Geometry check sheet. Reference: the model listing, model coordinates, mm. Face numbers are marked on the shaded views. A direction names the side the tool comes from. Coordinates: 2 decimals unless noted, no trailing zeros. Order: outer loops, then holes, each group sorted by start corner. A loop starts at its lowest first (then second) coordinate and runs counter-clockwise, first axis right, second up. Notation, with made-up numbers: (-22, 66) - (30, 66) arc R10 ccw to (30, 82) - close; hole circle Ø11 at (75, 57). An arc over 180 degrees is marked (long way). Return JSON: item names as keys, results as strings. Group by question number.
Item 1: Section check B-B on z = 51. Give the number of separate pieces and of enclosed holes in the cut face, then the cut area to 3 significant figures.
Item 2: Tool access check on the marked faces 1 and 2. Record the directions out of +Z, -Z, +X, -X, +Y, -Y that give a thin tool (end or side, any length) a straight path to the whole face; none if there is none.
Item 3: Section check A-A on y = 16.5. Enter the section's corners in (x, z) (3 decimals).
Item 4: Gauge pin test, flat ends, axial feed: pin 1 (1.6 mm diameter, centred on x = 36.5, y = 30, fed in from +Z); pin 2 (2.5 mm diameter, centred on x = 36.5, y = -8, fed in from +Z); pin 3 (1.5 mm diameter, centred on x = 8, y = -9.5, fed in from +Z) (3 decimals). Record the tip position at first contact, or that the pin passes through.
Item 5: Scan lines: probe 1 along X at (y, z) = (0.5, 11.5) (3 decimals); probe 2 along Z at (x, y) = (-19, -13) (3 decimals). Record each from-to range of solid material in increasing order.
Item 6: Section check C-C on x = -25.5. Enter the section's corners in (y, z) (3 decimals), then the cut area to 3 significant figures.
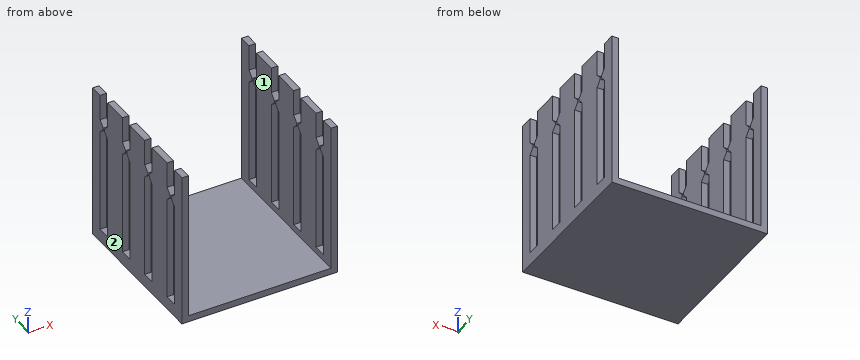
from build123d import *

# Parameters (mm, degrees)
F0_W     = 76.2
F0_H     = 76.2
F1_DEPTH = 76.2
F3_DEPTH = 131.88104
F4_W     = 69.85
F4_H     = 73.025
F5_DEPTH = 151.50575


with BuildPart() as f1:
    # F0 (on Top) → F1 (new body)
    with BuildSketch(Plane.XY):
        Rectangle(F0_W, F0_H)
    extrude(amount=F1_DEPTH)

    # F2 (on face) → F3 (cut)
    with BuildSketch(Plane.YZ.offset(38.1)):
        with BuildLine():
            Line((-25.4, 63.5), (-25.4, 76.2))
            Line((-25.4, 76.2), (-31.75, 76.2))
            Line((-31.75, 76.2), (-31.75, 63.5))
            Line((-31.75, 63.5), (-29.024013, 60.774013))
            ThreePointArc((-29.024013, 60.774013), (-29.21, 60.325), (-29.024013, 59.875987))
            Line((-29.024013, 59.875987), (-31.75, 57.15))
            Line((-31.75, 57.15), (-31.75, 6.35))
            Line((-31.75, 6.35), (-25.4, 6.35))
            Line((-25.4, 6.35), (-25.4, 57.15))
            Line((-25.4, 57.15), (-28.125987, 59.875987))
            ThreePointArc((-28.125987, 59.875987), (-27.94, 60.325), (-28.125987, 60.774013))
            Line((-28.125987, 60.774013), (-25.4, 63.5))
        make_face()
        with BuildLine():
            Line((-6.35, 63.5), (-6.35, 76.2))
            Line((-6.35, 76.2), (-12.7, 76.2))
            Line((-12.7, 76.2), (-12.7, 63.5))
            Line((-12.7, 63.5), (-9.974013, 60.774013))
            ThreePointArc((-9.974013, 60.774013), (-10.16, 60.325), (-9.974013, 59.875987))
            Line((-9.974013, 59.875987), (-12.7, 57.15))
            Line((-12.7, 57.15), (-12.7, 6.35))
            Line((-12.7, 6.35), (-6.35, 6.35))
            Line((-6.35, 6.35), (-6.35, 57.15))
            Line((-6.35, 57.15), (-9.075987, 59.875987))
            ThreePointArc((-9.075987, 59.875987), (-8.89, 60.325), (-9.075987, 60.774013))
            Line((-9.075987, 60.774013), (-6.35, 63.5))
        make_face()
        with BuildLine():
            Line((12.7, 76.2), (6.35, 76.2))
            Line((6.35, 76.2), (6.35, 63.5))
            Line((6.35, 63.5), (9.075987, 60.774013))
            ThreePointArc((9.075987, 60.774013), (8.89, 60.325), (9.075987, 59.875987))
            Line((9.075987, 59.875987), (6.35, 57.15))
            Line((6.35, 57.15), (6.35, 6.35))
            Line((6.35, 6.35), (12.7, 6.35))
            Line((12.7, 6.35), (12.7, 57.15))
            Line((12.7, 57.15), (9.974013, 59.875987))
            ThreePointArc((9.974013, 59.875987), (10.16, 60.325), (9.974013, 60.774013))
            Line((9.974013, 60.774013), (12.7, 63.5))
            Line((12.7, 63.5), (12.7, 76.2))
        make_face()
        with BuildLine():
            Line((31.75, 76.2), (25.4, 76.2))
            Line((25.4, 76.2), (25.4, 63.5))
            Line((25.4, 63.5), (28.125987, 60.774013))
            ThreePointArc((28.125987, 60.774013), (27.94, 60.325), (28.125987, 59.875987))
            Line((28.125987, 59.875987), (25.4, 57.15))
            Line((25.4, 57.15), (25.4, 6.35))
            Line((25.4, 6.35), (31.75, 6.35))
            Line((31.75, 6.35), (31.75, 57.15))
            Line((31.75, 57.15), (29.024013, 59.875987))
            ThreePointArc((29.024013, 59.875987), (29.21, 60.325), (29.024013, 60.774013))
            Line((29.024013, 60.774013), (31.75, 63.5))
            Line((31.75, 63.5), (31.75, 76.2))
        make_face()
        Polygon((-12.7, 76.2), (-6.35, 76.2), (6.35, 76.2), (12.7, 76.2), (25.4, 76.2), (31.75, 76.2), (31.627543, 85.504442), (-31.75, 85.504442), (-31.75, 76.2), (-25.4, 76.2), align=None)
    extrude(amount=-F3_DEPTH, mode=Mode.SUBTRACT)

    # F4 (on face) → F5 (cut)
    with BuildSketch(Plane.XZ.offset(38.1)):
        with Locations((0, 39.6875)):
            Rectangle(F4_W, F4_H)
    extrude(amount=-F5_DEPTH, mode=Mode.SUBTRACT)


solid = f1.part
Computed:
{
 "1": {"separate pieces": "10", "enclosed holes": "0", "area": "323 mm²"},
 "2": {"face 1": "+Z, +Y, -Y", "face 2": "+Z, -Z, -X, +Y, -Y"},
 "3": {"outline": "(-38.1, 0) - (38.1, 0) - (38.1, 76.2) - (34.925, 76.2) - (34.925, 3.175) - (-34.925, 3.175) - (-34.925, 76.2) - (-38.1, 76.2) - close"},
 "4": {"pin 1": "stops at z = 62.55", "pin 2": "stops at z = 63.1", "pin 3": "stops at z = 3.175"},
 "5": {"probe 1": "x = -38.1 to -34.925, 34.925 to 38.1", "probe 2": "z = 0 to 3.175"},
 "6": {"outline": "(-38.1, 0) - (38.1, 0) - (38.1, 3.175) - (-38.1, 3.175) - close", "area": "242 mm²"}
}
